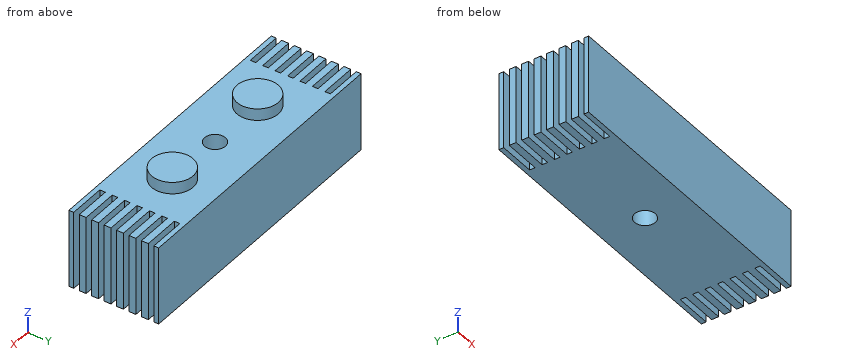
```python
from build123d import *

# Parameters (mm, degrees)
F0_W     = 42
F0_H     = 13
F1_DEPTH = 13
F2_W     = 42
F2_H     = 13
F2_R     = 3
F3_DEPTH = 1.7
F4_W     = 5.5
F4_H     = 0.8
F5_DEPTH = 11.301
F7_R     = 1.5
F8_DEPTH = 11.301


with BuildPart() as f1:
    # F0 (on Top) → F1 (new body)
    with BuildSketch(Plane.XY):
        Rectangle(F0_W, F0_H)
    extrude(amount=F1_DEPTH)

    # F2 (on face) → F3 (cut)
    with BuildSketch(Plane.XY.offset(13)):
        Rectangle(F2_W, F2_H)
        with Locations((-8.85, 0)):
            Circle(F2_R, mode=Mode.SUBTRACT)
        with Locations((8.85, 0)):
            Circle(F2_R, mode=Mode.SUBTRACT)
    extrude(amount=-F3_DEPTH, mode=Mode.SUBTRACT)

    # F4 (on face) → F5 (cut, through all)
    with BuildSketch(Plane.XY.offset(11.3)):
        with Locations((18.35, 5.4)):
            Rectangle(F4_W, F4_H)
        with Locations((18.35, 3.6)):
            Rectangle(F4_W, F4_H)
        with Locations((18.35, 1.8)):
            Rectangle(F4_W, F4_H)
        with Locations((18.35, 0)):
            Rectangle(F4_W, F4_H)
        with Locations((18.35, -1.8)):
            Rectangle(F4_W, F4_H)
        with Locations((18.35, -3.6)):
            Rectangle(F4_W, F4_H)
        with Locations((18.35, -5.4)):
            Rectangle(F4_W, F4_H)
        with Locations((-18.380066, 5.4)):
            Rectangle(F4_W, F4_H)
        with Locations((-18.380066, 3.6)):
            Rectangle(F4_W, F4_H)
        with Locations((-18.380066, 1.8)):
            Rectangle(F4_W, F4_H)
        with Locations((-18.380066, 0)):
            Rectangle(F4_W, F4_H)
        with Locations((-18.380066, -1.8)):
            Rectangle(F4_W, F4_H)
        with Locations((-18.380066, -3.6)):
            Rectangle(F4_W, F4_H)
        with Locations((-18.380066, -5.4)):
            Rectangle(F4_W, F4_H)
    extrude(amount=-F5_DEPTH, mode=Mode.SUBTRACT)

    # F7 (on face) → F8 (cut, through all)
    with BuildSketch(Plane.XY.offset(11.3)):
        Circle(F7_R)
    extrude(amount=-F8_DEPTH, mode=Mode.SUBTRACT)


solid = f1.part
```
Geometry check sheet. Reference: the model listing, model coordinates, mm. Coordinates: 2 decimals unless noted, no trailing zeros. Order: outer loops, then holes, each group sorted by start corner. A loop starts at its lowest first (then second) coordinate and runs counter-clockwise, first axis right, second up. Notation, with made-up numbers: (78.5, -35) - (104.5, -35) arc R19 ccw to (104.5, -18) - close; hole circle Ø1 at (-6.75, 65). An arc over 180 degrees is marked (long way). Answer as a JSON object with one key per item and string values. Group by question number.
Item 1: Sectioned sample at A-A, the plane x = -18. Give the number of separate pieces and of enclosed holes in the cut face, and give its area (3 significant figures).
Item 2: Sectioned sample at C-C, the plane x = 0. Record the cut outline in (y, z).
Item 3: Scan lines: probe 1 along Y at (x, z) = (0, 3.75); probe 2 along Z at (x, y) = (-3.5, -1.25); probe 3 along X at (y, z) = (-1, 1.75). Record each from-to range of solid material in increasing order.
Item 4: Sectioned sample at D-D, the plane x = 8.85. Record the cut outline in (y, z), and give its area (3 significant figures).
Item 5: Sectioned sample at B-B, the plane y = 0. Record the cut outline in (x, z).
Resolved:
{
 "1": {"separate pieces": "8", "enclosed holes": "0", "area": "83.6 mm^2"},
 "2": {"outline": "(-6.5, 0) - (-1.5, 0) - (-1.5, 11.3) - (-6.5, 11.3) - close; (1.5, 0) - (6.5, 0) - (6.5, 11.3) - (1.5, 11.3) - close"},
 "3": {"probe 1": "-6.5 to -1.5, 1.5 to 6.5", "probe 2": "0 to 11.3", "probe 3": "-21 to -1.12, 1.12 to 21"},
 "4": {"outline": "(-6.5, 0) - (6.5, 0) - (6.5, 11.3) - (3, 11.3) - (3, 13) - (-3, 13) - (-3, 11.3) - (-6.5, 11.3) - close", "area": "157 mm^2"},
 "5": {"outline": "(-15.63, 0) - (-1.5, 0) - (-1.5, 11.3) - (-5.85, 11.3) - (-5.85, 13) - (-11.85, 13) - (-11.85, 11.3) - (-15.63, 11.3) - close; (1.5, 0) - (15.6, 0) - (15.6, 11.3) - (11.85, 11.3) - (11.85, 13) - (5.85, 13) - (5.85, 11.3) - (1.5, 11.3) - close"}
}
